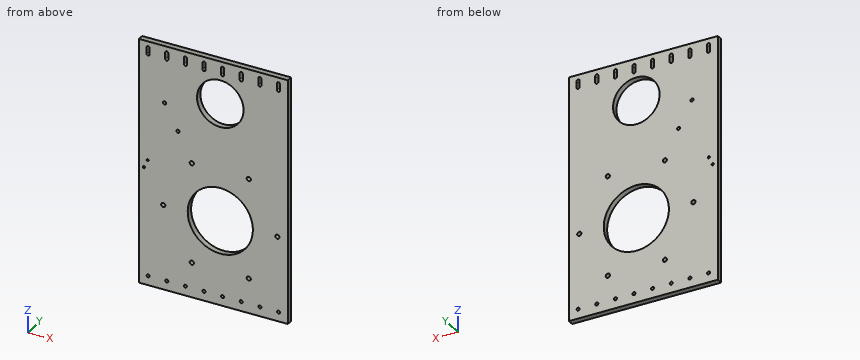
from build123d import *

# Parameters (mm, degrees)
SKETCH1_W           = 160
SKETCH1_H           = 260
SKETCH1_R           = 35
SKETCH1_R_2         = 25
SKETCH1_R_3         = 2.25
SKETCH1_R_4         = 1.175
SKETCH1_R_5         = 1.65
BOSS_EXTRUDE1_DEPTH = 6.35
SKETCH2_R           = 1.7
CUT_EXTRUDE1_DEPTH  = 306.352783678


with BuildPart() as part:
    # Sketch1 → Boss-Extrude1 (new body)
    with BuildSketch(Plane(origin=(0, 0, 0), x_dir=(1, 0, 0), z_dir=(0, 1, 0))):
        with Locations((80, 130)):
            Rectangle(SKETCH1_W, SKETCH1_H)
        with Locations(Location((87.5, 170, 0), (0, 0, 270))):
            Circle(SKETCH1_R, mode=Mode.SUBTRACT)
        with Locations(Location((87.5, 45, 0), (0, 0, 270))):
            Circle(SKETCH1_R_2, mode=Mode.SUBTRACT)
        with Locations(Location((148.75, 170, 0), (0, 0, 270))):
            Circle(SKETCH1_R_3, mode=Mode.SUBTRACT)
        with Locations(Location((118.125, 116.955944018, 0), (0, 0, 270))):
            Circle(SKETCH1_R_3, mode=Mode.SUBTRACT)
        with Locations(Location((56.875, 116.955944018, 0), (0, 0, 270))):
            Circle(SKETCH1_R_3, mode=Mode.SUBTRACT)
        with Locations(Location((26.25, 170, 0), (0, 0, 270))):
            Circle(SKETCH1_R_3, mode=Mode.SUBTRACT)
        with Locations(Location((56.875, 223.044055982, 0), (0, 0, 270))):
            Circle(SKETCH1_R_3, mode=Mode.SUBTRACT)
        with Locations(Location((118.125, 223.044055982, 0), (0, 0, 270))):
            Circle(SKETCH1_R_3, mode=Mode.SUBTRACT)
        with Locations(Location((5.475532842, 135.298909731, 0), (0, 0, 270))):
            Circle(SKETCH1_R_4, mode=Mode.SUBTRACT)
        with Locations(Location((9.516263037, 126.701090269, 0), (0, 0, 270))):
            Circle(SKETCH1_R_4, mode=Mode.SUBTRACT)
        with Locations(Location((10, 250, 0), (0, 0, 270))):
            Circle(SKETCH1_R_5, mode=Mode.SUBTRACT)
        with Locations(Location((30, 250, 0), (0, 0, 270))):
            Circle(SKETCH1_R_5, mode=Mode.SUBTRACT)
        with Locations(Location((50, 250, 0), (0, 0, 270))):
            Circle(SKETCH1_R_5, mode=Mode.SUBTRACT)
        with Locations(Location((70, 250, 0), (0, 0, 270))):
            Circle(SKETCH1_R_5, mode=Mode.SUBTRACT)
        with Locations(Location((90, 250, 0), (0, 0, 270))):
            Circle(SKETCH1_R_5, mode=Mode.SUBTRACT)
        with Locations(Location((110, 250, 0), (0, 0, 270))):
            Circle(SKETCH1_R_5, mode=Mode.SUBTRACT)
        with Locations(Location((130, 250, 0), (0, 0, 270))):
            Circle(SKETCH1_R_5, mode=Mode.SUBTRACT)
        with Locations(Location((150, 250, 0), (0, 0, 270))):
            Circle(SKETCH1_R_5, mode=Mode.SUBTRACT)
        with BuildLine():
            Line((8.35, 6.5), (8.35, 13.5))
            ThreePointArc((8.35, 13.5), (10, 15.15), (11.65, 13.5))
            Line((11.65, 13.5), (11.65, 6.5))
            ThreePointArc((11.65, 6.5), (10, 4.85), (8.35, 6.5))
        make_face(mode=Mode.SUBTRACT)
        with BuildLine():
            Line((31.65, 6.5), (31.65, 13.5))
            ThreePointArc((31.65, 13.5), (30, 15.15), (28.35, 13.5))
            Line((28.35, 13.5), (28.35, 6.5))
            ThreePointArc((28.35, 6.5), (30, 4.85), (31.65, 6.5))
        make_face(mode=Mode.SUBTRACT)
        with BuildLine():
            Line((51.65, 6.5), (51.65, 13.5))
            ThreePointArc((51.65, 13.5), (50, 15.15), (48.35, 13.5))
            Line((48.35, 13.5), (48.35, 6.5))
            ThreePointArc((48.35, 6.5), (50, 4.85), (51.65, 6.5))
        make_face(mode=Mode.SUBTRACT)
        with BuildLine():
            Line((71.65, 6.5), (71.65, 13.5))
            ThreePointArc((71.65, 13.5), (70, 15.15), (68.35, 13.5))
            Line((68.35, 13.5), (68.35, 6.5))
            ThreePointArc((68.35, 6.5), (70, 4.85), (71.65, 6.5))
        make_face(mode=Mode.SUBTRACT)
        with BuildLine():
            Line((91.65, 6.5), (91.65, 13.5))
            ThreePointArc((91.65, 13.5), (90, 15.15), (88.35, 13.5))
            Line((88.35, 13.5), (88.35, 6.5))
            ThreePointArc((88.35, 6.5), (90, 4.85), (91.65, 6.5))
        make_face(mode=Mode.SUBTRACT)
        with BuildLine():
            Line((111.65, 6.5), (111.65, 13.5))
            ThreePointArc((111.65, 13.5), (110, 15.15), (108.35, 13.5))
            Line((108.35, 13.5), (108.35, 6.5))
            ThreePointArc((108.35, 6.5), (110, 4.85), (111.65, 6.5))
        make_face(mode=Mode.SUBTRACT)
        with BuildLine():
            Line((131.65, 6.5), (131.65, 13.5))
            ThreePointArc((131.65, 13.5), (130, 15.15), (128.35, 13.5))
            Line((128.35, 13.5), (128.35, 6.5))
            ThreePointArc((128.35, 6.5), (130, 4.85), (131.65, 6.5))
        make_face(mode=Mode.SUBTRACT)
        with BuildLine():
            Line((151.65, 6.5), (151.65, 13.5))
            ThreePointArc((151.65, 13.5), (150, 15.15), (148.35, 13.5))
            Line((148.35, 13.5), (148.35, 6.5))
            ThreePointArc((148.35, 6.5), (150, 4.85), (151.65, 6.5))
        make_face(mode=Mode.SUBTRACT)
    extrude(amount=BOSS_EXTRUDE1_DEPTH)

    # Sketch2 → Cut-Extrude1 (cut, through all)
    with BuildSketch(Plane(origin=(0, 6.35, 0), x_dir=(1, 0, 0), z_dir=(0, 1, 0))):
        with Locations(Location((27.663890721, 60.64097268, 0), (0, 0, 270))):
            Circle(SKETCH2_R)
        with Locations(Location((42.063890721, 86.95902732, 0), (0, 0, 270))):
            Circle(SKETCH2_R)
    extrude(amount=-CUT_EXTRUDE1_DEPTH, mode=Mode.SUBTRACT)


solid = part.part
Here's how the part is built. I have some questions about the finished solid (model axes, mm). Round coordinates to 2 decimals unless told otherwise and drop trailing zeros. Loops run counter-clockwise (first coordinate to the right, second up) from the corner with the lowest first, then second, coordinate; pieces in that order, holes last.
1. If we section it at B-B on y = 4: Count the separate pieces of the cut face and the enclosed holes in it, plus the area to 3 significant figures.
Answer list:
separate pieces: 1
enclosed holes: 28
area: 35,300 mm2
2. If we section it at A-A on z = -144.5: Write out the boundary of the cut face in (x, y), plus the area to 3 significant figures.
Answer list:
outline: (0, 0) - (63.53, 0) - (63.53, 6.35) - (0, 6.35) - close; (111.47, 0) - (160, 0) - (160, 6.35) - (111.47, 6.35) - close
area: 712 mm2
3. For P1, Ø3, axis at x = 70, z = -250, coming from the +Y side; P2, Ø5.5, axis at x = 150, z = -250, coming from the -Y side, each with a flat end and sliding along its axis, tell me the tip position at first contact or that it passes through.
Answer list:
P1: passes through
P2: stops at y = 0
4. If I drill on line 1 along Z through (x, y) = (91, 0.75); line 2 along Z through (x, y) = (49, 1.25); line 3 along Z through (x, y) = (90.5, 2.75), over which ranges is the centre line in solid material (lowest first)?
Answer list:
line 1: z = -260 to -251.31, -248.69 to -204.82, -135.18 to -69.75, -20.25 to -14.81, -5.19 to 0
line 2: z = -260 to -251.31, -248.69 to -14.81, -5.19 to 0
line 3: z = -260 to -251.57, -248.43 to -204.87, -135.13 to -69.82, -20.18 to -15.07, -4.93 to 0
